Answer from the drawing. Dimensions are ordinates in mm from the lowest x, y and z of the part. Give positions to 0.01 mm unless a question says otherwise; leave off trailing zeros. Loops run counter-clockwise (first coordinate to the right, second up) from the corner with the lowest first, then second, coordinate; pieces in that order, holes last. Notation, with made-up numbers: (-27.5, 18) - (28.5, 18) arc R12 ccw to (28.5, 22) - close; hole circle Ø2 at (-23.75, 49.5). An arc over 180 degrees is marked (long way). Put each result on its own line as item: value. Start each with the question number.
1. A cutting plane is placed at C-C, the plane x = 47. Determine the outline of the cut face in (y, z).
2. A cutting plane is placed at D-D, the plane y = 52.5. Determine the outline of the cut face in (x, z).
3. Given pin 1 Ø4.5 at (y, z) = (30, 3.5) entering from +X; pin 2 Ø2.5 at (x, z) = (56, 4.5) entering from +Y; pin 3 Ø5 at (x, z) = (32, 2.5) entering from -Y, each flat-ended and moving along its own axis, determine where each tip first touches the part or whether it passes through.
4. For a pull along X with two mould halves and no side action, classify the marked faces 1, 2 and 3 as released by +X, released by -X, zero draft, split by the parting line, or undercut.
5. A cutting plane is placed at B-B, the plane z = 2. Determine the outline of the cut face in (x, y).
6. Consider L1, parallel to Y at x = 49, z = 4.5; L2, parallel to X at y = 20, z = 5.75; L3, parallel to X at y = 12, z = 5. Determine where each line is inside the solid, lowest interval first. Write a range as from..to.
7. A cutting plane is placed at A-A, the plane y = 38. Determine the outline of the cut face in (x, z), plus the area to 3 significant figures.
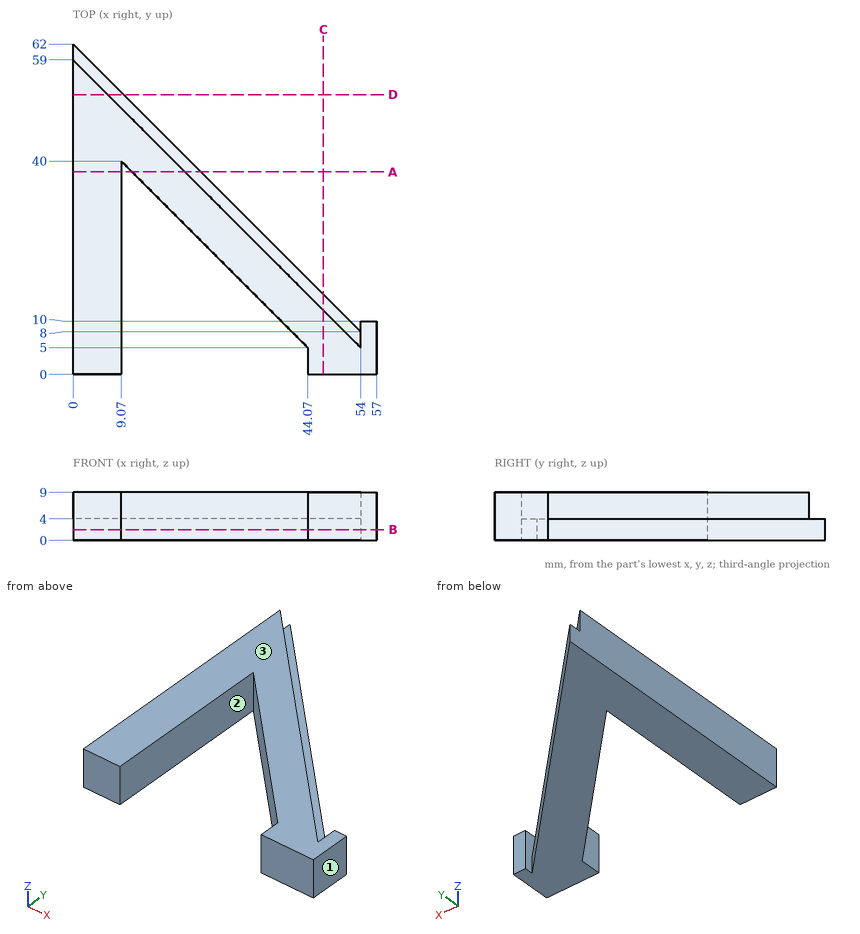
Return value:
1. outline: (0, 0) - (15, 0) - (15, 4) - (12, 4) - (12, 9) - (0, 9) - close
2. outline: (0, 0) - (9.5, 0) - (9.5, 4) - (6.5, 4) - (6.5, 9) - (0, 9) - close
3. pin 1: stops at x = 34.25
3. pin 2: stops at y = 10
3. pin 3: stops at y = 14.57
4. face 1: released by +X
4. face 2: undercut
4. face 3: zero draft
5. outline: (0, 0) - (9.07, 0) - (9.07, 40) - (44.07, 5) - (44.07, 0) - (57, 0) - (57, 10) - (54, 10) - (54, 8) - (0, 62) - close
6. L1: y = 0..10
6. L2: x = 0..9.07, 29.07..39
6. L3: x = 0..9.07, 37.07..47
7. outline: (0, 0) - (9.07, 0) - (9.07, 9) - (0, 9) - close; (11.07, 0) - (24, 0) - (24, 4) - (21, 4) - (21, 9) - (11.07, 9) - close
7. area: 183 mm2
